Here's how the part is built. I have some questions about the finished solid (model axes, mm). A direction names the side the tool comes from. Round coordinates to 2 decimals unless told otherwise and drop trailing zeros. Write each loop counter-clockwise with the first axis right and the second up, starting at its lowest first coordinate (ties: lowest second). Pieces come first, ordered by that corner, then holes. Notation, with made-up numbers: (-9, 60.25) - (39, 60.25) arc R14 ccw to (39, 77.25) - close; hole circle Ø1 at (55, -40). An arc over 180 degrees is marked (long way). Return JSON: item names as keys, results as strings. Group by question number.
Autodesk Inventor part; units mm, degrees
ref_plane "作業平面1" through (0, -415, 0) normal (0, 1, 0) x (-1, 0, 0)
ref_plane "YZ Plane" through (0, 0, 0) normal (1, 0, 0) x (0, 1, 0)
ref_plane "XY Plane" through (0, 0, 0) normal (0, 0, 1) x (1, 0, 0)
sketch "スケッチ1" plane through (0, 0, 0) normal (1, 0, 0) x (0, 1, 0)
  line L0 (-700, 210) -> (-700, 490)
  line L1 (-700, 490) -> (-400, 690)
  line L2 (-400, 690) -> (-250, 690)
  line L3 (-250, 690) -> (0, 150)
  line L4 (0, 150) -> (0, 0)
  line L5 (0, 0) -> (-230, 0)
  arc A0 (-230, 0) -> (-700, 210) centre (-700, -420.9524) ccw
  dimension "d0" = 690
  dimension "d1" = 280
  dimension "d2" = 200
  dimension "d3" = 300
  dimension "d4" = 150
  dimension "d5" = 700
  dimension "d6" = 230
  dimension "d7" = 150
extrude "押し出し1" add sketch "スケッチ1" along normal blind 5
sketch "スケッチ2" plane through (5, 0, 0) normal (1, 0, 0) x (0, 0, -1)
  circle A0 centre (-100, -87) radius 2.5
  line L0 (0, 0) -> (-150, 0)
  line L1 (0, -230) -> (0, 0)
  circle A1 centre (-125, -164) radius 2.5
  dimension "d10" = 87
  dimension "d11" = 100
  dimension "d12" = 5
  dimension "d13" = 164
  dimension "d14" = 125
  dimension "d15" = 5
extrude "押し出し2" cut sketch "スケッチ2" against normal through all
ref_plane "作業平面1" through (0, -415, 0) normal (0, 1, 0) x (-1, 0, 0)
sketch "スケッチ6" plane through (0, -415, 0) normal (0, 1, 0) x (-1, 0, 0)
  line L0 (-10, 590) -> (-5, 575)
  line L1 (-10, 575) -> (-5, 560)
  line L2 (-5, 150) -> (-5, 690)
  line L3 (-10, 575) -> (-5.5, 576.5)
  line L4 (-10, 590) -> (-5, 591.6667)
  point P0 (0, 0)
  dimension "d48" = 15
  dimension "d55" = 15
  dimension "d56" = 15
extrude "押し出し6" add sketch "スケッチ6" against normal blind 120
sketch "スケッチ7" plane through (5, -535, 591.6667) normal (0.3162, 0, 0.9487) x (0.9487, 0, -0.3162)
  line L0 (0, 0) -> (0, 120)
  line L1 (0, 118) -> (3.2705, 118)
  line L2 (3.2705, 118) -> (3.2705, 2)
  line L3 (3.2705, 2) -> (0, 2)
  line L4 (0, 2) -> (0, 118)
  line L5 (5.2705, 120) -> (5.2705, 0)
  line L6 (5.2705, 118) -> (8.0139, 118)
  line L7 (8.0139, 118) -> (8.0139, 2)
  line L8 (8.0139, 2) -> (5.2705, 2)
  line L9 (5.2705, 2) -> (5.2705, 118)
  line L10 (5.2705, 0) -> (0, 0)
  line L11 (10.0139, 120) -> (10.0139, 0)
  line L12 (0, 120) -> (5.2705, 120)
  point P0 (182.358, 535)
  dimension "d57" = 2
  dimension "d58" = 2
  dimension "d59" = 2
  dimension "d60" = 2
extrude "押し出し7" cut sketch "スケッチ7" against normal through all contours L0 L1 L2 L3 | L5 L6 L7 L8
equation "\"d59\" = d58"
properties part number "end_plate" material "CFRP"
1) Imagine slicing it at A-A (y = -493). Give the number of separate pieces and of enclosed holes in the cut face, plus the area to 3 significant figures.
2) If we mould it in two halves opening along X, with no side actions, what happens to faces 1 (the flat face through (5, -355, 350)), 2 (the flat face through (2.535, -475.812, 584.271)), 3 (the flat face through (2.5, -552.1, 588.6))? For each: released by +X, released by -X, zero draft, split by the parting line, or undercut.
3) Will these pins go through, and if not, where does the flat tip stop? pin 1 Ø2 at (x, z) = (2, 98) entering from -Y; pin 2 Ø1 at (y, z) = (-86.5, 165) entering from +X; pin 3 Ø2.5 at (x, z) = (8.5, 573) entering from +Y; pin 4 Ø2.5 at (x, z) = (7.5, 578) entering from -Y.
4) Imagine slicing it at D-D (z = 275.5). Please give me the cut outline in (x, y).
5) For faces 4 (the flat face through (2.8, -474.2, 568.4)), 5 (the cylindrical face through (2.465, -446.003, 156.617)), which set-ups out of +Z, -Z, +X, -X, +Y, -Y let a thin tool reach every point of the face, with its end or its side?
6) Imagine slicing it at B-B (x = 2.5). Please give me the cut outline in (y, z).
7) I need wall thicknesses on line 1 along X through (y, z) = (-545, 374.5); line 2 along Z through (x, y) = (2.65, -164); line 3 along Y through (x, z) = (3.25, 125). Which ranges of each line are inside material? Lowest first, please.
8) Imagine slicing it at C-C (z = 163.5). Please give me the cut outline in (x, y).
Results found:
{
 "1": {"separate pieces": "3", "enclosed holes": "0", "area": "2,220 mm²"},
 "2": {"face 1": "released by +X", "face 2": "undercut", "face 3": "zero draft"},
 "3": {"pin 1": "stops at y = -342.58", "pin 2": "stops at x = 5", "pin 3": "stops at y = -415", "pin 4": "passes through"},
 "4": {"outline": "(0, -700) - (5, -700) - (5, -58.1) - (0, -58.1) - close"},
 "5": {"face 4": "none", "face 5": "-Z, +X, -X, -Y"},
 "6": {"outline": "(-700, 210) arc R630.95 cw to (-230, 0) - (0, 0) - (0, 150) - (-250, 690) - (-400, 690) - (-700, 490) - close; hole (-533, 558.82) - (-417, 558.82) - (-417, 567.5) - (-533, 567.5) - close; hole (-533, 573.82) - (-417, 573.82) - (-417, 584.17) - (-533, 584.17) - close; hole circle Ø5 at (-164, 125); hole circle Ø5 at (-87, 100)"},
 "7": {"line 1": "x = 0 to 5", "line 2": "z = 0 to 122.5, 127.5 to 504.24", "line 3": "y = -383.71 to -166.5, -161.5 to 0"},
 "8": {"outline": "(0, -462.27) - (5, -462.27) - (5, -6.25) - (0, -6.25) - close"}
}
